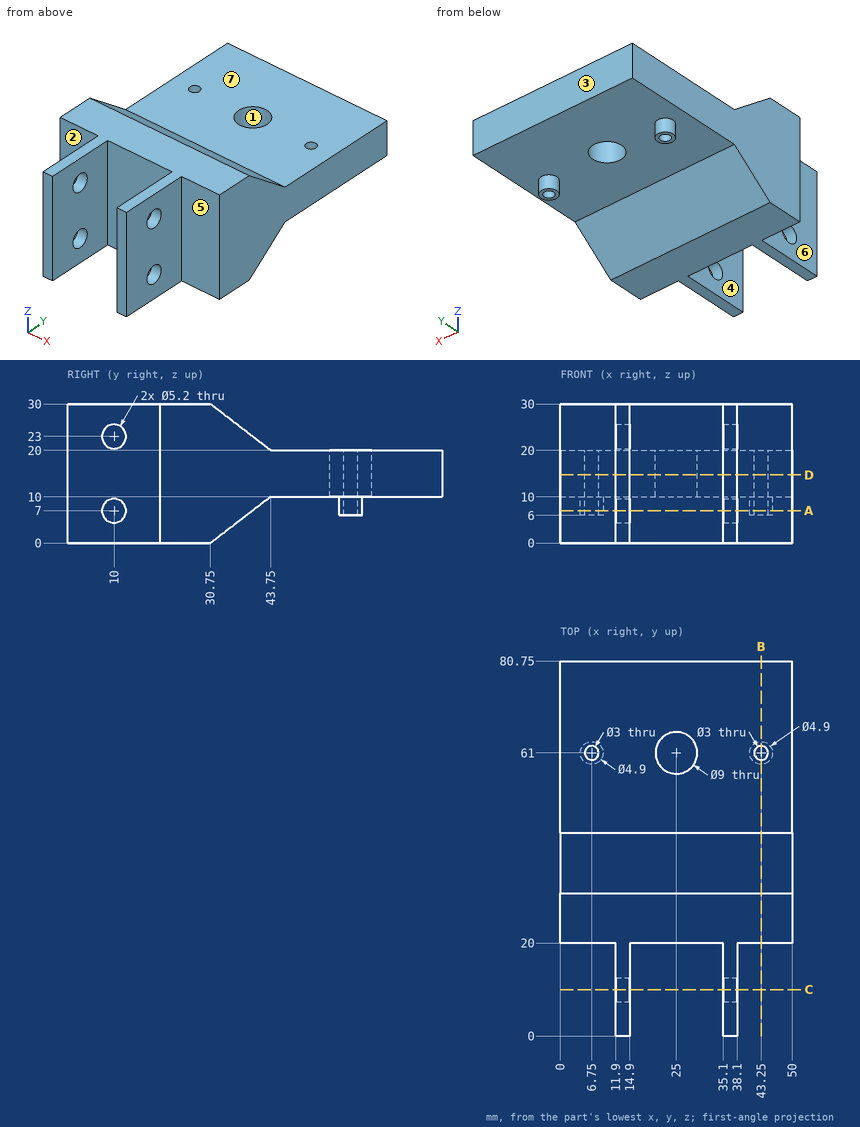
Here's the drawing with two shaded views (mm, measured from the low corner). I have some questions. A direction names the side the tool comes from. Coordinates: 2 decimals unless noted, no trailing zeros. Loops run counter-clockwise (first coordinate to the right, second up) from the corner with the lowest first, then second, coordinate; pieces in that order, holes last. Notation, with made-up numbers: (52, 16.5) -> (75, 16.5) arc R21 ccw to (75, 22.5) -> close; hole circle Ø3 at (52, -34.75). An arc over 180 degrees is marked (long way). Answer in a Markdown table with one row per item.
(1) Imagine slicing it at B-B (x = 43.25). List the corners of the cut face in (y, z) for me.
Results found:
| item | result |
|---|---|
| outline | (20, 0) -> (30.75, 0) -> (43.75, 10) -> (58.55, 10) -> (58.55, 6) -> (59.5, 6) -> (59.5, 20) -> (43.75, 20) -> (30.75, 30) -> (20, 30) -> close; (62.5, 6) -> (63.45, 6) -> (63.45, 10) -> (80.75, 10) -> (80.75, 20) -> (62.5, 20) -> close |
(2) Imagine slicing it at D-D (z = 14.75). List the corners of the cut face in (x, y) for me.
Results found:
| item | result |
|---|---|
| outline | (0, 20) -> (11.9, 20) -> (11.9, 0) -> (14.9, 0) -> (14.9, 20) -> (35.1, 20) -> (35.1, 0) -> (38.1, 0) -> (38.1, 20) -> (50, 20) -> (50, 80.75) -> (0, 80.75) -> close; hole circle Ø3 at (6.75, 61); hole circle Ø9 at (25, 61); hole circle Ø3 at (43.25, 61) |
(3) Imagine slicing it at C-C (y = 10). List the corners of the cut face in (x, z) for me, plus the area to 3 significant figures.
Results found:
| item | result |
|---|---|
| outline | (11.9, 0) -> (14.9, 0) -> (14.9, 4.4) -> (11.9, 4.4) -> close; (11.9, 9.6) -> (14.9, 9.6) -> (14.9, 20.4) -> (11.9, 20.4) -> close; (11.9, 25.6) -> (14.9, 25.6) -> (14.9, 30) -> (11.9, 30) -> close; (35.1, 0) -> (38.1, 0) -> (38.1, 4.4) -> (35.1, 4.4) -> close; (35.1, 9.6) -> (38.1, 9.6) -> (38.1, 20.4) -> (35.1, 20.4) -> close; (35.1, 25.6) -> (38.1, 25.6) -> (38.1, 30) -> (35.1, 30) -> close |
| area | 118 mm^2 |
(4) If I drill on probe 1 along X at (y, z) = (18.5, 17); probe 2 along Z at (x, y) = (12, 10.5); probe 3 along Y at (x, z) = (33, 19.5), over which ranges is the centre line in solid material (lowest first)?
Results found:
| item | result |
|---|---|
| probe 1 | x = 11.9 to 14.9, 35.1 to 38.1 |
| probe 2 | z = 0 to 4.45, 9.55 to 20.45, 25.55 to 30 |
| probe 3 | y = 20 to 80.75 |
(5) Thinking about a two-plate mould opening in Y: for the marked faces 1, 2 and 3, which applies, released by +Y, released by -Y, zero draft, split by the parting line, or undercut?
Results found:
| item | result |
|---|---|
| face 1 | undercut |
| face 2 | released by -Y |
| face 3 | released by +Y |
(6) Imagine slicing it at A-A (z = 7). List the corners of the cut face in (x, y) for me, plus the area to 3 significant figures.
Results found:
| item | result |
|---|---|
| outline | (0, 20) -> (11.9, 20) -> (11.9, 12.6) -> (14.9, 12.6) -> (14.9, 20) -> (35.1, 20) -> (35.1, 12.6) -> (38.1, 12.6) -> (38.1, 20) -> (50, 20) -> (50, 39.85) -> (0, 39.85) -> close; circle Ø4.9 at (6.75, 61); (11.9, 0) -> (14.9, 0) -> (14.9, 7.4) -> (11.9, 7.4) -> close; (35.1, 0) -> (38.1, 0) -> (38.1, 7.4) -> (35.1, 7.4) -> close; circle Ø4.9 at (43.25, 61); hole circle Ø3 at (6.75, 61); hole circle Ø3 at (43.25, 61) |
| area | 1,100 mm^2 |
(7) For the marked faces 4, 5, 6 and 7, which set-ups out of +Z, -Z, +X, -X, +Y, -Y let a thin tool reach every point of the face, with its end or its side?
Results found:
| item | result |
|---|---|
| face 4 | +Z, -Z, -Y |
| face 5 | +Z, -Z, +X, -Y |
| face 6 | +Z, -Z, -X, -Y |
| face 7 | +Z, +X, -X, +Y |
(8) Will these pins go through, and if not, where does the flat tip stop? pin 1 Ø3.5 at (x, z) = (44.5, 21) entering from -Y; pin 2 Ø5 at (x, z) = (34.5, 15) entering from -Y; pin 3 Ø16 at (y, z) = (8.5, 22.5) entering from -X; pin 4 Ø2 at (x, z) = (9.5, 22) entering from +Y.
Results found:
| item | result |
|---|---|
| pin 1 | stops at y = 20 |
| pin 2 | stops at y = 0 |
| pin 3 | stops at x = 11.9 |
| pin 4 | stops at y = 42.45 |
